```python
from build123d import *

# Parameters (mm, degrees)
F2_DEPTH = 10.16
F3_R     = 3.89255
F4_DEPTH = 1.27
F5_R     = 2.36855
F6_DEPTH = 6.096
F8_DEPTH = 1.65


with BuildPart() as f2:
    # F1 (on Top) → F2 (new body)
    with BuildSketch(Plane.XY):
        with BuildLine():
            Line((-11.5060112064, -1.0844146426), (-9.3802938474, -1.6539988923))
            ThreePointArc((-9.3802938474, -1.6539988923), (9.525, 0), (-9.3802938474, 1.6539988923))
            Line((-9.3802938474, 1.6539988923), (-11.5060112064, 1.0844146426))
            ThreePointArc((-11.5060112064, 1.0844146426), (-11.557, 0), (-11.5060112064, -1.0844146426))
        make_face()
    extrude(amount=F2_DEPTH)

    # F3 (on face) → F4 (join)
    with BuildSketch(Plane.XY.offset(10.16)):
        Circle(F3_R)
    extrude(amount=F4_DEPTH)

    # F5 (on face) → F6 (cut)
    with BuildSketch(Plane.XY.offset(11.43)):
        Circle(F5_R)
    extrude(amount=-F6_DEPTH, mode=Mode.SUBTRACT)

    # F7 (on face) → F8 (join)
    with BuildSketch(Plane.XY.offset(5.334)):
        with BuildLine():
            ThreePointArc((0.55, 2.3038075229), (0, 2.36855), (-0.55, 2.3038075229))
            Line((-0.55, 2.3038075229), (-0.55, 1.0099504938))
            ThreePointArc((-0.55, 1.0099504938), (-1.15, 0), (-0.55, -1.0099504938))
            Line((-0.55, -1.0099504938), (-0.55, -2.3038075229))
            ThreePointArc((-0.55, -2.3038075229), (0, -2.36855), (0.55, -2.3038075229))
            Line((0.55, -2.3038075229), (0.55, -1.0099504938))
            ThreePointArc((0.55, -1.0099504938), (1.15, 0), (0.55, 1.0099504938))
            Line((0.55, 1.0099504938), (0.55, 2.3038075229))
        make_face()
    extrude(amount=F8_DEPTH)


solid = f2.part
```
CAD build for the part. Positions are in the model's coordinates, mm. A direction names the side the tool comes from. Round coordinates to 2 decimals unless told otherwise and drop trailing zeros. Loops run counter-clockwise (first coordinate to the right, second up) from the corner with the lowest first, then second, coordinate; pieces in that order, holes last. Notation, with made-up numbers: (78.5, 40) - (108.5, 40) arc R26 ccw to (108.5, 56) - close; hole circle Ø8 at (-19.5, 28.5). An arc over 180 degrees is marked (long way). Return JSON: item names as keys, results as strings. Group by question number.
Q1. Band-saw the part on A-A on z = 6.5. Give the cut face in (x, y) (3 decimals).
Q2. Band-saw the part on C-C on x = 0. Give the cut face in (y, z) (3 decimals).
Q3. Drill centre lines: line 1 along Y through (x, z) = (0, 8.5) (3 decimals); line 2 along Z through (x, y) = (2.25, 4); line 3 along X through (y, z) = (1, 7.75). Where is each one in solid material? Low to high. Write a range as [from, to].
Q4. Flat gauge pins, fed straight in: pin 1 Ø1 at (y, z) = (-2, 6) entering from +X; pin 2 Ø0.7 at (x, y) = (0, -0.5) entering from +Z; pin 3 Ø1 at (x, z) = (-8.5, 4.5) entering from +Y. Where does each tip first touch, or does it go through?
Q5. Two-plate mould, pull along X, no slides. Class faces 3 (the face through (-0.84, -3.8, 10.79)), 4 (the face through (-11.557, 0.015, 5.009)), 5 (the face through (-0.55, -2, 6)): +X half, -X half, draft (parallel to the pull), parting line (faces both ways), or undercut.
Q6. Band-saw the part on B-B on y = 0. Give the cut face in (x, z) (3 decimals).
Q7. Tool access for faces 1 (the face through (2, -2, 11.43)), 2 (the face through (-0.55, 2, 6)): list every direction of +Z, -Z, +X, -X, +Y, -Y with a clear straight run to the whole face (end or side of a thin tool).
Q8. Band-saw the part on D-D on z = 1.75. Give the cut face in (x, y) (3 decimals).
Solutions:
{
 "1": {"outline": "(-11.506, -1.084) - (-9.38, -1.654) arc R9.525 ccw (long way) to (-9.38, 1.654) - (-11.506, 1.084) arc R11.557 ccw to start; hole (-0.55, -2.304) - (-0.55, -1.01) arc R1.15 cw to (-0.55, 1.01) - (-0.55, 2.304) arc R2.369 ccw to start; hole (0.55, -2.304) arc R2.369 ccw to (0.55, 2.304) - (0.55, 1.01) arc R1.15 cw to (0.55, -1.01) - close"},
 "2": {"outline": "(-9.525, 0) - (9.525, 0) - (9.525, 10.16) - (3.893, 10.16) - (3.893, 11.43) - (2.369, 11.43) - (2.369, 6.984) - (-2.369, 6.984) - (-2.369, 11.43) - (-3.893, 11.43) - (-3.893, 10.16) - (-9.525, 10.16) - close"},
 "3": {"line 1": "y = [-9.525, -2.369], [2.369, 9.525]", "line 2": "z = [0, 10.16]", "line 3": "x = [-11.51, -2.15], [2.15, 9.47]"},
 "4": {"pin 1": "stops at x = 9.41", "pin 2": "stops at z = 6.98", "pin 3": "stops at y = 5.17"},
 "5": {"face 3": "parting line", "face 4": "-X half", "face 5": "undercut"},
 "6": {"outline": "(-11.557, 0) - (9.525, 0) - (9.525, 10.16) - (3.893, 10.16) - (3.893, 11.43) - (2.369, 11.43) - (2.369, 5.334) - (1.15, 5.334) - (1.15, 6.984) - (-1.15, 6.984) - (-1.15, 5.334) - (-2.369, 5.334) - (-2.369, 11.43) - (-3.893, 11.43) - (-3.893, 10.16) - (-11.557, 10.16) - close"},
 "7": {"face 1": "+Z, +X, -X, +Y, -Y", "face 2": "+Z"},
 "8": {"outline": "(-11.506, -1.084) - (-9.38, -1.654) arc R9.525 ccw (long way) to (-9.38, 1.654) - (-11.506, 1.084) arc R11.557 ccw to start"}
}
